Geometry check sheet. Reference: the model listing, model coordinates, mm. Face numbers are marked on the shaded views. A direction names the side the tool comes from. Round coordinates to 2 decimals unless told otherwise and drop trailing zeros. Write each loop counter-clockwise with the first axis right and the second up, starting at its lowest first coordinate (ties: lowest second). Pieces come first, ordered by that corner, then holes. Notation, with made-up numbers: (3.25, 26.25) - (32.25, 26.25) arc R31 cw to (32.25, 53.25) - close; hole circle Ø2 at (44, -6.75). An arc over 180 degrees is marked (long way). One line per question, with ' | ' between items. Start each with the question number.
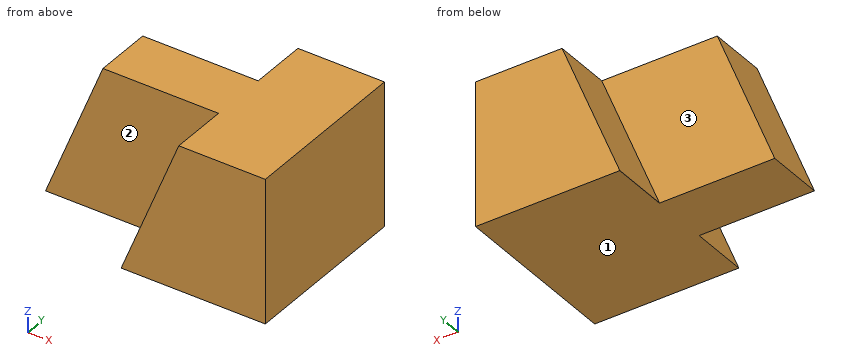
from build123d import *

# Parameters (mm, degrees)
F0_W      = 57.15
F0_H      = 31.75
F1_DEPTH  = 38.1
F3_DEPTH  = 64.77
F4_W      = 12.7
F4_H      = 32.225172
F5_DEPTH  = 25.4
F7_DEPTH  = 12.7
F9_DEPTH  = 12.7
F11_DEPTH = 12.7


with BuildPart() as f1:
    # F0 (on Front) → F1 (new body)
    with BuildSketch(Plane.XZ):
        with Locations((28.575, 15.875)):
            Rectangle(F0_W, F0_H)
    extrude(amount=F1_DEPTH)

    # F2 (on Front) → F3 (cut)
    with BuildSketch(Plane.XZ):
        Polygon((0, 0), (12.7, 31.884328), (0, 31.884328), align=None)
    extrude(amount=F3_DEPTH, mode=Mode.SUBTRACT)

    # F4 (on Right) → F5 (cut)
    with BuildSketch(Plane.YZ):
        with Locations((-6.35, 16.112586)):
            Rectangle(F4_W, F4_H)
        Polygon((-25.4, 0), (-25.4, 32.225172), (-38.1, 32.225172), (-38.209904, 0), align=None)
    extrude(amount=F5_DEPTH, mode=Mode.SUBTRACT)

    # F6 (on Front) → F7 (cut)
    with BuildSketch(Plane.XZ):
        Polygon((38.103979, 31.787962), (25.397928, 31.787962), (25.365233, 0), align=None)
    extrude(amount=F7_DEPTH, mode=Mode.SUBTRACT)

    # F8 (on Front) → F9 (cut)
    with BuildSketch(Plane.XZ):
        Polygon((75.160764, -53.294525), (61.148994, -53.294525), (61.104827, -85.576326), (79.001695, -128.796339), (79.001695, -96.281484), (93.439646, -96.281484), align=None)
        Polygon((94.494686, -128.999516), (93.439646, -96.281484), (79.001695, -96.281484), (79.001695, -128.796339), align=None)
    extrude(amount=-F9_DEPTH, mode=Mode.SUBTRACT)

    # F10 (on face) → F11 (cut)
    with BuildSketch(Plane.XZ.offset(38.1)):
        Polygon((25.4, 0), (38.1, 31.75), (25.4, 31.75), align=None)
    extrude(amount=-F11_DEPTH, mode=Mode.SUBTRACT)


solid = f1.part
Q1. Go/stop test with flat-tipped pins: P1, Ø1, axis at x = 35, y = -27.5, coming from the -Z side; P2, Ø9.5, axis at x = 19, z = 16, coming from the +Y side. Record where each tip stops, or that it passes through.
Q2. Section check C-C, the plane x = 18. Record the cut outline in (y, z), then the cut area to 3 significant figures.
Q3. Thickness scan on line 1 (Y direction, x = 32, z = 24); line 2 (X direction, y = -30, z = 8); line 3 (X direction, y = -25.5, z = 23). Record the ranges inside material, lowest first.
Q4. Section check B-B, the plane y = -6. Record the cut outline in (x, z), then the cut area to 3 significant figures.
Q5. Section check A-A, the plane z = 18. Record the cut outline in (x, y).
Q6. Section check D-D, the plane z = 29. Record the cut outline in (x, y).
Q7. Set-up check for the marked faces 1, 2 and 3: record each of +Z, -Z, +X, -X, +Y, -Y from which the full face is reachable in a straight line by a thin tool's end or side.
Result sheet:
1) P1: z = 0 | P2: y = -12.7
2) outline: (-25.4, 0) - (-12.7, 0) - (-12.7, 31.75) - (-25.4, 31.75) - close | area: 403 mm²
3) line 1: -25.4 to -12.7 | line 2: 28.6 to 57.15 | line 3: 34.6 to 57.15
4) outline: (25.4, 0) - (57.15, 0) - (57.15, 31.75) - (38.09, 31.75) - (25.4, 0.09) - close | area: 807 mm²
5) outline: (7.17, -25.4) - (32.6, -25.4) - (32.6, -38.1) - (57.15, -38.1) - (57.15, 0) - (32.58, 0) - (32.58, -12.7) - (7.17, -12.7) - close
6) outline: (11.55, -25.4) - (37, -25.4) - (37, -38.1) - (57.15, -38.1) - (57.15, 0) - (36.99, 0) - (36.99, -12.7) - (11.55, -12.7) - close
7) face 1: -Z, +X, -X, +Y, -Y | face 2: +Z, -X, -Y | face 3: +Z, -X, +Y
